from build123d import *

# Parameters (mm, degrees)
SKETCH1_R           = 30
BOSS_EXTRUDE1_DEPTH = 40
BOSS_EXTRUDE2_DEPTH = 20
SKETCH4_R           = 7
CUT_EXTRUDE2_DEPTH  = 84.713798146
SKETCH2_R           = 25
CUT_EXTRUDE1_DEPTH  = 95.910484142


with BuildPart() as part:
    # Sketch1 → Boss-Extrude1 (new body)
    with BuildSketch(Plane(origin=(0, 0, 0), x_dir=(1, 0, 0), z_dir=(0, 1, 0))):
        with Locations(Location((0, 0, 0), (0, 0, 270))):
            Circle(SKETCH1_R)
    extrude(amount=BOSS_EXTRUDE1_DEPTH)

    # Sketch3 → Boss-Extrude2 (add)
    with BuildSketch(Plane.XZ):
        with BuildLine():
            ThreePointArc((-48.485281374, -31.514718626), (-48.485281374, -48.485281374), (-31.514718626, -48.485281374))
            ThreePointArc((-31.514718626, -48.485281374), (0, -41.542775524), (31.514718626, -48.485281374))
            ThreePointArc((31.514718626, -48.485281374), (48.485281374, -48.485281374), (48.485281374, -31.514718626))
            ThreePointArc((48.485281374, -31.514718626), (41.542775524, 0), (48.485281374, 31.514718626))
            ThreePointArc((48.485281374, 31.514718626), (48.485281374, 48.485281374), (31.514718626, 48.485281374))
            ThreePointArc((31.514718626, 48.485281374), (0, 41.542775524), (-31.514718626, 48.485281374))
            ThreePointArc((-31.514718626, 48.485281374), (-48.485281374, 48.485281374), (-48.485281374, 31.514718626))
            ThreePointArc((-48.485281374, 31.514718626), (-41.542775524, 0), (-48.485281374, -31.514718626))
        make_face()
    extrude(amount=BOSS_EXTRUDE2_DEPTH)

    # Sketch4 → Cut-Extrude2 (cut, through all)
    with BuildSketch(Plane(origin=(0, 0, 0), x_dir=(1, 0, 0), z_dir=(0, 1, 0))):
        with Locations(Location((-40, 40, 0), (0, 0, 270))):
            Circle(SKETCH4_R)
        with Locations(Location((40, -40, 0), (0, 0, 270))):
            Circle(SKETCH4_R)
        with Locations(Location((40, 40, 0), (0, 0, 270))):
            Circle(SKETCH4_R)
        with Locations(Location((-40, -40, 0), (0, 0, 270))):
            Circle(SKETCH4_R)
    extrude(amount=-CUT_EXTRUDE2_DEPTH, mode=Mode.SUBTRACT)

    # Sketch2 → Cut-Extrude1 (cut, through all)
    with BuildSketch(Plane(origin=(0, 40, 0), x_dir=(1, 0, 0), z_dir=(0, 1, 0))):
        with Locations(Location((0, 0, 0), (0, 0, 270))):
            Circle(SKETCH2_R)
    extrude(amount=-CUT_EXTRUDE1_DEPTH, mode=Mode.SUBTRACT)


solid = part.part
Source: CAD feature listing. Evaluate the final solid. Frame: model axes, mm. Round coordinates to 2 decimals unless told otherwise and drop trailing zeros. Loops run counter-clockwise (first coordinate to the right, second up) from the corner with the lowest first, then second, coordinate; pieces in that order, holes last. Notation, with made-up numbers: M 45.5,-27.5 L 99.5,-27.5 A15 cw 99.5,-9.5 Z; hole C -25.75,-27 d3. An arc over 180 degrees is marked long. Return JSON: item names as keys, results as strings. Group by question number.
1. Section query C-C on z = -40. Output: boundary loops of the cut face in (x, y).
2. Section query B-B on x = 0. Output: boundary loops of the cut face in (y, z), and give its area (3 significant figures).
3. Material intervals for line 1 along X through (y, z) = (-5.25, -40); line 2 along Z through (x, y) = (37, -3); line 3 along Z through (x, y) = (39, -2), sorted ascending. Write a range as from..to.
4. Section query D-D on y = -13.5. Output: boundary loops of the cut face in (x, z), and give its area (3 significant figures).
5. Section query A-A on z = 0. Output: boundary loops of the cut face in (x, y), and give its area (3 significant figures).
6. Mould query, pull axis Z, two halves, no side actions, for faces 1 (the face through (1.32, 19.72, -29.97)), 2 (the face through (-0.455, -9.86, -41.544)), 3 (the face through (22, 0, -22)), 4 (the face through (-41.544, -9.86, 0.455)). Classes: released by +Z, released by -Z, zero draft, split by the parting line, or undercut.
7. Pin query (flat end, axial travel): pin 1 (2 mm diameter, centred on x = 11, z = 39.5, fed in from +Y); pin 2 (11 mm diameter, centred on x = -40, z = 40, fed in from -Y); pin 3 (8 mm diameter, centred on y = 16, z = 28, fed in from +X); pin 4 (12 mm diameter, centred on y = -8.5, z = 12, fed in from -X). Return the tip coordinate at first contact, or that it passes through.
Checks:
{
 "1": {"outline": "M -52,-20 L -47,-20 L -47,0 L -52,0 Z; M -33,-20 L 33,-20 L 33,0 L -33,0 Z; M 47,-20 L 52,-20 L 52,0 L 47,0 Z"},
 "2": {"outline": "M -20,-41.54 L 0,-41.54 L 0,-30 L 40,-30 L 40,-25 L -20,-25 Z; M -20,25 L 40,25 L 40,30 L 0,30 L 0,41.54 L -20,41.54 Z", "area": "1,060 mm²"},
 "3": {"line 1": "x = -52..-47, -33..33, 47..52", "line 2": "z = -51.62..-46.32, -33.68..33.68, 46.32..51.62", "line 3": "z = -51.96..-46.93, -33.07..33.07, 46.93..51.96"},
 "4": {"outline": "M -48.49,-31.51 A12 ccw -31.51,-48.49 A75 cw 31.51,-48.49 A12 ccw 48.49,-31.51 A75 cw 48.49,31.51 A12 ccw 31.51,48.49 A75 cw -31.51,48.49 A12 ccw -48.49,31.51 A75 cw Z; hole C -40,-40 d14; hole C -40,40 d14; hole C 0,0 d50; hole C 40,-40 d14; hole C 40,40 d14", "area": "5,970 mm²"},
 "5": {"outline": "M -41.54,-20 L -25,-20 L -25,40 L -30,40 L -30,0 L -41.54,0 Z; M 25,-20 L 41.54,-20 L 41.54,0 L 30,0 L 30,40 L 25,40 Z", "area": "1,060 mm²"},
 "6": {"face 1": "split by the parting line", "face 2": "released by -Z", "face 3": "zero draft", "face 4": "undercut"},
 "7": {"pin 1": "stops at y = 0", "pin 2": "passes through", "pin 3": "stops at x = 18", "pin 4": "stops at x = -43.73"}
}
